```python
from build123d import *

# Parameters (mm, degrees)
SKETCH1_W               = 50.8
SKETCH1_H               = 25.4
SKETCH1_W_2             = 45.72
SKETCH1_H_2             = 20.32
BOSS_EXTRUDE1_DEPTH     = 355.6
F_8_CLEARANCE_HOLE1_D   = 4.4958
F_1_1_DIAMETER_HOLE1_D  = 25.4
SKETCH8_W               = 50.8
SKETCH8_H               = 50.8
CUT_EXTRUDE1_DEPTH      = 421.64
CUT_EXTRUDE1_DEPTH_BACK = 71.882


with BuildPart() as part:
    # Sketch1 → Boss-Extrude1 (new body)
    with BuildSketch(Plane.XY):
        Rectangle(SKETCH1_W, SKETCH1_H)
        Rectangle(SKETCH1_W_2, SKETCH1_H_2, mode=Mode.SUBTRACT)
    extrude(amount=-BOSS_EXTRUDE1_DEPTH)

    # #8 Clearance Hole1 (through all)
    with Locations(Plane(origin=(25.4, 0, 0), x_dir=(0, 0, -1), z_dir=(1, 0, 0))):
        with Locations((12.7, 0), (38.1, 0), (63.5, 0), (88.9, 0), (114.3, 0), (139.7, 0), (165.1, 0), (190.5, 0), (215.9, 0), (241.3, 0), (266.7, 0), (292.1, 0), (317.5, 0), (342.9, 0)):
            Hole(F_8_CLEARANCE_HOLE1_D / 2)

    # 1 (1) Diameter Hole1 (through all)
    with Locations(Plane(origin=(0, 12.7, 0), x_dir=(1, 0, 0), z_dir=(0, 1, 0))):
        with Locations((0, 101.6)):
            Hole(F_1_1_DIAMETER_HOLE1_D / 2)

    # Sketch8 → Cut-Extrude1 (cut, two sides)
    with BuildSketch(Plane(origin=(0, 12.7, 0), x_dir=(1, 0, 0), z_dir=(0, 1, 0))) as cut_extrude1_sk:
        with Locations((0, 25.4)):
            Rectangle(SKETCH8_W, SKETCH8_H)
    extrude(amount=CUT_EXTRUDE1_DEPTH, mode=Mode.SUBTRACT)
    extrude(cut_extrude1_sk.sketch, amount=-CUT_EXTRUDE1_DEPTH_BACK, mode=Mode.SUBTRACT)


solid = part.part
```
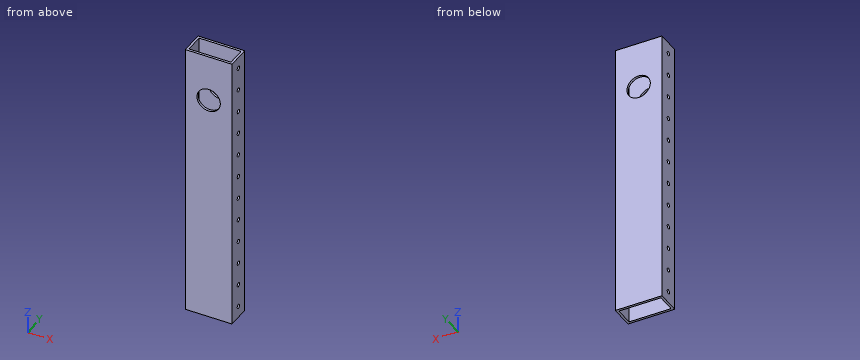
Check sheet for the modelled part. Datum: model origin and axes. Units: mm. Round coordinates to 2 decimals unless told otherwise and drop trailing zeros. Loops run counter-clockwise (first coordinate to the right, second up) from the corner with the lowest first, then second, coordinate; pieces in that order, holes last. Notation, with made-up numbers: (56.25, 61) -> (65.25, 61) arc R37 ccw to (65.25, 100) -> close; hole circle Ø10 at (-34.75, 78). An arc over 180 degrees is marked (long way). Answer in a Markdown table with one row per item.
Q1. Sectioned sample at A-A on z = -101.6. Enter the section's corners in (x, y), then the cut area to 3 significant figures.
Data:
| item | result |
|---|---|
| outline | (-25.4, -12.7) -> (-12.7, -12.7) -> (-12.7, -10.16) -> (-22.86, -10.16) -> (-22.86, 10.16) -> (-12.7, 10.16) -> (-12.7, 12.7) -> (-25.4, 12.7) -> close; (12.7, -12.7) -> (25.4, -12.7) -> (25.4, 12.7) -> (12.7, 12.7) -> (12.7, 10.16) -> (22.86, 10.16) -> (22.86, -10.16) -> (12.7, -10.16) -> close |
| area | 232 mm^2 |
Q2. Sectioned sample at C-C on x = 0. Enter the section's corners in (y, z).
Data:
| item | result |
|---|---|
| outline | (-12.7, -355.6) -> (-10.16, -355.6) -> (-10.16, -114.3) -> (-12.7, -114.3) -> close; (-12.7, -88.9) -> (-10.16, -88.9) -> (-10.16, -50.8) -> (-12.7, -50.8) -> close; (10.16, -355.6) -> (12.7, -355.6) -> (12.7, -114.3) -> (10.16, -114.3) -> close; (10.16, -88.9) -> (12.7, -88.9) -> (12.7, -50.8) -> (10.16, -50.8) -> close |
Q3. Go/stop test with a flat-tipped pin: P1, Ø7, axis at y = 0, z = -215.9, coming from the -X side. Record where the tip stops, or that it passes through.
Data:
| item | result |
|---|---|
| P1 | stops at x = -25.4 |
Q4. Sectioned sample at D-D on y = -7.5. Enter the section's corners in (x, z), then the cut area to 3 significant figures.
Data:
| item | result |
|---|---|
| outline | (-25.4, -355.6) -> (-22.86, -355.6) -> (-22.86, -50.8) -> (-25.4, -50.8) -> close; (22.86, -355.6) -> (25.4, -355.6) -> (25.4, -50.8) -> (22.86, -50.8) -> close |
| area | 1,550 mm^2 |
Q5. Thickness scan on L1, parallel to Y at x = 24.1, z = -190.5; L2, parallel to Y at x = -19, z = -86; L3, parallel to X at y = 0, z = -172. Record the ranges inside material, lowest first.
Data:
| item | result |
|---|---|
| L1 | y = -12.7 to -2.25, 2.25 to 12.7 |
| L2 | y = -12.7 to -10.16, 10.16 to 12.7 |
| L3 | x = -25.4 to -22.86, 22.86 to 25.4 |
Q6. Sectioned sample at B-B on x = 19. Enter the section's corners in (y, z), then the cut area to 3 significant figures.
Data:
| item | result |
|---|---|
| outline | (-12.7, -355.6) -> (-10.16, -355.6) -> (-10.16, -50.8) -> (-12.7, -50.8) -> close; (10.16, -355.6) -> (12.7, -355.6) -> (12.7, -50.8) -> (10.16, -50.8) -> close |
| area | 1,550 mm^2 |
